from build123d import *

# Parameters (mm, degrees)
SKETCH1_W               = 457.2
SKETCH1_H               = 840.74
BOSS_EXTRUDE1_DEPTH     = 1.2192
SKETCH5_W               = 27.94
SKETCH5_H               = 241.3
CUT_EXTRUDE1_DEPTH      = 1.2192
F_1_4_CLEARANCE_HOLE2_D = 6.7564


with BuildPart() as part:
    # Sketch1 → Boss-Extrude1 (new body)
    with BuildSketch(Plane.XY):
        with Locations((228.6, 420.37)):
            Rectangle(SKETCH1_W, SKETCH1_H)
    extrude(amount=BOSS_EXTRUDE1_DEPTH)

    # Sketch5 → Cut-Extrude1 (cut)
    with BuildSketch(Plane.XY.offset(1.2192)):
        with Locations((13.97, 690.88)):
            Rectangle(SKETCH5_W, SKETCH5_H)
        Polygon((457.2, 840.74), (0, 840.74), (0, 811.53), (27.94, 811.53), (429.26, 811.53), (457.2, 811.53), align=None)
        with Locations((443.23, 690.88)):
            Rectangle(SKETCH5_W, SKETCH5_H)
    extrude(amount=-CUT_EXTRUDE1_DEPTH, mode=Mode.SUBTRACT)

    # 1/4 Clearance Hole2 (through all)
    with Locations(Plane.XY.offset(1.2192)):
        with Locations((50.8, 798.83), (228.6, 798.83), (406.4, 798.83), (12.7, 532.13), (12.7, 265.43), (12.7, 24.13), (444.5, 24.13), (444.5, 265.43), (444.5, 532.13)):
            Hole(F_1_4_CLEARANCE_HOLE2_D / 2)


solid = part.part
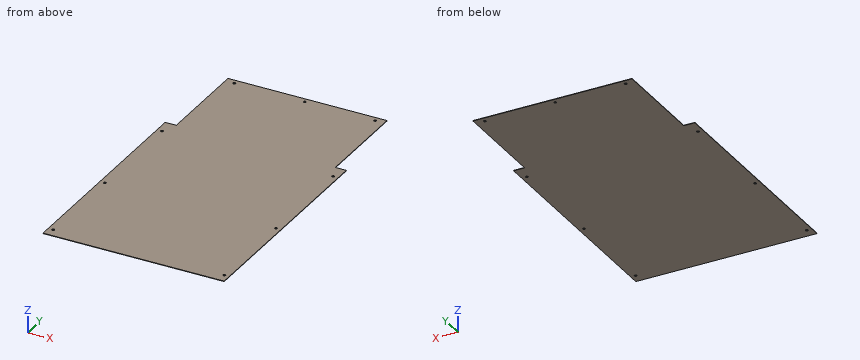
Design review of the part built by this model. Coordinates are the model's own, in mm. Give positions to 0.01 mm unless a question says otherwise; leave off trailing zeros. Loops run counter-clockwise (first coordinate to the right, second up) from the corner with the lowest first, then second, coordinate; pieces in that order, holes last. Notation, with made-up numbers: M -8.75,35.5 L 33.25,35.5 A20 cw 33.25,71.5 Z; hole C 57.25,75.5 d10. An arc over 180 degrees is marked long. One line per question, with ' | ' between items. Start each with the question number.
1. Add section A-A (z = 0.8). Give the number of separate pieces and of enclosed holes in the cut face, plus the area to 3 significant figures.
2. Add section B-B (y = 744). Write out the cut boundary in (x, z).
3. Insertion check: P1, Ø5.5, axis at x = 12.7, y = 265.43, coming from the -Z side; P2, Ø0.6, axis at x = 16, z = 0.5, coming from the +Y side. Each pin has a flat end and moves straight along its axis. Give the tip position at first contact, or say it passes through.
4. To check wall thickness, follow L1, parallel to Y at x = 12.7, z = 0.4; L2, parallel to X at y = 798.83, z = 0.9; L3, parallel to X at y = 532.13, z = 0.6. State the ranges of each line that lie inside material, in increasing order.
Worked out:
1) separate pieces: 1 | enclosed holes: 9 | area: 357,000 mm²
2) outline: M 27.94,0 L 429.26,0 L 429.26,1.22 L 27.94,1.22 Z
3) P1: passes through | P2: stops at y = 570.23
4) L1: y = 0 to 20.75, 27.51 to 262.05, 268.81 to 528.75, 535.51 to 570.23 | L2: x = 27.94 to 47.42, 54.18 to 225.22, 231.98 to 403.02, 409.78 to 429.26 | L3: x = 0 to 9.32, 16.08 to 441.12, 447.88 to 457.2
